```python
from build123d import *

# Parameters (mm, degrees)
SKETCH1_R           = 1.5
BOSS_EXTRUDE1_DEPTH = 4
CHAMFER1_SIZE       = 2
CHAMFER2_SIZE       = 1.55


with BuildPart() as part:
    # Sketch1 → Boss-Extrude1 (new body)
    with BuildSketch(Plane(origin=(0, 0, 0), x_dir=(1, 0, 0), z_dir=(0, 1, 0))):
        Polygon((0, 0), (110.6, 0), (118.6, 0), (118.6, 8), (110.6, 8), (110.6, 80), (118.6, 80), (118.6, 88), (110.6, 88), (110.6, 160), (118.6, 160), (118.6, 168), (110.6, 168), (0, 168), (-8, 168), (-8, 160), (0, 160), (0, 88), (-8, 88), (-8, 80), (0, 80), (0, 8), (-8, 8), (-8, 0), align=None)
        with Locations(Location((114.6, 164, 0), (0, 0, 270))):
            Circle(SKETCH1_R, mode=Mode.SUBTRACT)
        with Locations(Location((114.6, 84, 0), (0, 0, 90))):
            Circle(SKETCH1_R, mode=Mode.SUBTRACT)
        with Locations(Location((114.6, 4, 0), (0, 0, 270))):
            Circle(SKETCH1_R, mode=Mode.SUBTRACT)
        with Locations(Location((-4, 4, 0), (0, 0, 90))):
            Circle(SKETCH1_R, mode=Mode.SUBTRACT)
        with Locations(Location((-4, 84, 0), (0, 0, 270))):
            Circle(SKETCH1_R, mode=Mode.SUBTRACT)
        with Locations(Location((-4, 164, 0), (0, 0, 90))):
            Circle(SKETCH1_R, mode=Mode.SUBTRACT)
    extrude(amount=BOSS_EXTRUDE1_DEPTH)

    # Chamfer1
    chamfer1_edges = [part.edges().sort_by_distance(p)[0] for p in [
        (-8, 2, 0),
        (-8, 2, -8),
        (0, 2, -8),
        (0, 2, -80),
        (-8, 2, -80),
        (-8, 2, -88),
        (0, 2, -88),
        (0, 2, -160),
        (-8, 2, -160),
        (-8, 2, -168),
        (118.6, 2, -168),
        (118.6, 2, -160),
        (110.6, 2, -160),
        (110.6, 2, -88),
        (118.6, 2, -88),
        (118.6, 2, -80),
        (110.6, 2, -80),
        (110.6, 2, -8),
        (118.6, 2, -8),
        (118.6, 2, 0),
    ]]
    chamfer(chamfer1_edges, length=CHAMFER1_SIZE)

    # Chamfer2
    chamfer2_edges = [part.edges().sort_by_distance(p)[0] for p in [
        (114.6, 4, -165.5),
        (114.6, 4, -82.5),
        (114.6, 4, -5.5),
        (-4, 4, -2.5),
        (-4, 4, -85.5),
        (-4, 4, -162.5),
    ]]
    chamfer(chamfer2_edges, length=CHAMFER2_SIZE)


solid = part.part
```
Build history of the part. All positions in model axes, mm. A direction names the side the tool comes from. Round coordinates to 2 decimals unless told otherwise and drop trailing zeros. Write each loop counter-clockwise with the first axis right and the second up, starting at its lowest first coordinate (ties: lowest second). Pieces come first, ordered by that corner, then holes.
1) Band-saw the part on A-A, the plane y = 0.8. Give the number of separate pieces and of enclosed holes in the cut face, and give its area (3 significant figures).
2) Band-saw the part on B-B, the plane z = -117.5. List the corners of the cut face in (x, y), and give its area (3 significant figures).
3) Drill centre lines: probe 1 along X at (y, z) = (1.3, -4); probe 2 along Z at (x, y) = (114.6, 0.65); probe 3 along X at (y, z) = (0.2, -85). Where is each one in solid material? Low to high.
4) 3-axis set-ups, long thin cutter, end or side, ignore diameter. For faces 1 (the flat face through (-4, 2, -8)), 2 (the flat face through (115, 2, -80)), 3 (the flat face through (-8, 2, -4)): which of +Z, -Z, +X, -X, +Y, -Y reach the whole face in a straight line?
5) Pin check, flat tips, straight feed: pin 1 (2.5 mm diameter, centred on x = 114.6, z = -4, fed in from +Y); pin 2 (1.2 mm diameter, centred on y = 2, z = -113, fed in from +X). Stop position of each tip, or through.
Ans:
1. separate pieces: 1
1. enclosed holes: 6
1. area: 18,900 mm2
2. outline: (0, 0) - (110.6, 0) - (110.6, 4) - (0, 4) - close
2. area: 442 mm2
3. probe 1: x = -8 to -5.5, -2.5 to 113.1, 116.1 to 118.6
3. probe 2: z = -168 to -165.5, -162.5 to -160, -88 to -85.5, -82.5 to -80, -8 to -5.5, -2.5 to 0
3. probe 3: x = -8 to -5.12, -2.88 to 113.48, 115.72 to 118.6
4. face 1: -X, +Y, -Y
4. face 2: +X, +Y, -Y
4. face 3: +Z, -Z, -X, +Y, -Y
5. pin 1: passes through
5. pin 2: stops at x = 110.6
